```python
from build123d import *

# Parameters (mm, degrees)
F0_R          = 2.3
F1_DEPTH      = 13
F3_DEPTH      = 46
F6_DEPTH      = 52.2
F8_DEPTH      = 25
F10_DEPTH     = 25
F11_T1_DEPTH  = 69.4664340584
F11_T3_DEPTH  = 69.4664340584
F11_T8_DEPTH  = 31.9524083705
F11_T13_DEPTH = 31.9524083705
F11_T19_DEPTH = 31.9524083705
F11_T23_DEPTH = 31.9524083705
F15_DEPTH     = 4
F16_DEPTH     = 4
F19_DEPTH     = 28
F20_R         = 2.3
F21_DEPTH     = 25
F22_R         = 2.3
F23_DEPTH     = 25
F24_R         = 0.5


# Not quite as in the source:
# - a fillet or chamfer that OpenCascade refuses, or shapes differently, is made with other operations: its cross-section is extruded or revolved along the edge and cut away or added
# - a feature names something its author has since deleted; it is built from what else it names


with BuildPart() as f1:
    # F0 (on Front) → F1 (new body)
    with BuildSketch(Plane.XZ):
        Polygon((10, 40), (-10, 40), (-17.9806351662, -11.8325809017), (-8.0368565166, -18.5498173996), (0, -8.6111112242), (8.0368565166, -18.5498173996), (17.9806351662, -11.8325809017), align=None)
        with Locations((-12, 0)):
            Circle(F0_R, mode=Mode.SUBTRACT)
        with Locations((12, 0)):
            Circle(F0_R, mode=Mode.SUBTRACT)
    extrude(amount=-F1_DEPTH)

    # F2 (on face) → F3 (cut)
    with BuildSketch(Plane.XY.offset(40)):
        with BuildLine():
            Line((-8, 0), (8, 0))
            ThreePointArc((8, 0), (0, 8), (-8, 0))
        make_face()
    extrude(amount=-F3_DEPTH, mode=Mode.SUBTRACT)

    # F5 (on offset) → F6 (cut)
    with BuildSketch(Plane.YZ.offset(25)):
        Polygon((13, -3.9485500787), (4.1381944902, -18.5498173996), (13, -18.5498173996), align=None)
    extrude(amount=-F6_DEPTH, mode=Mode.SUBTRACT)

    # F7 (on face) → F8 (cut)
    with BuildSketch(Plane(origin=(-11.122658813, 0, -16.4652915326), x_dir=(0.8286482208, 0, -0.5597697082), z_dir=(-0.5597697082, 0, -0.8286482208))):
        with BuildLine():
            ThreePointArc((-6.8761009811, 0), (-2.2761009811, -4.6), (2.3238990189, 0))
            Line((2.3238990189, 0), (-6.8761009811, 0))
        make_face()
    extrude(amount=-F8_DEPTH, mode=Mode.SUBTRACT)

    # F9 (on face) → F10 (cut)
    with BuildSketch(Plane(origin=(11.122658813, 0, -16.4652915326), x_dir=(0.8286482208, 0, 0.5597697082), z_dir=(0.5597697082, 0, -0.8286482208))):
        with BuildLine():
            ThreePointArc((-2.3238990189, 0), (2.2761009811, -4.6), (6.8761009811, 0))
            Line((6.8761009811, 0), (-2.3238990189, 0))
        make_face()
    extrude(amount=-F10_DEPTH, mode=Mode.SUBTRACT)

    # F11: fillet of radius 5 on 4 edges, made by hand

    # F11_s2 → F11_t1 (cut)
    with BuildSketch(Plane(origin=(7.6867833124, 0, 49.9240736631), x_dir=(0, 1, 0), z_dir=(-0.152176248, 0, -0.9883533728))):
        with BuildLine():
            ThreePointArc((13, -10.9705836466), (11.5355339059, -14.5061175525), (8, -15.9705836466))
            Line((8, -15.9705836466), (13, -15.9705836466))
            Line((13, -15.9705836466), (13, -10.9705836466))
        make_face()
    extrude(amount=F11_T1_DEPTH, mode=Mode.SUBTRACT)

    # F11_s4 → F11_t3 (cut)
    with BuildSketch(Plane(origin=(2.8843579817, 0, -18.733310736), x_dir=(0, 1, 0), z_dir=(-0.152176248, 0, 0.9883533728))):
        with BuildLine():
            ThreePointArc((8, -15.9705836466), (11.5355339059, -14.5061175525), (13, -10.9705836466))
            Line((13, -10.9705836466), (13, -15.9705836466))
            Line((13, -15.9705836466), (8, -15.9705836466))
        make_face()
    extrude(amount=F11_T3_DEPTH, mode=Mode.SUBTRACT)


with BuildPart() as f11_tool6:
    # F11_s7 → F11_t8 (new body)
    with BuildSketch(Plane(origin=(4.0911710208, 3.0705977915, 5.0593097692), x_dir=(0.6002776597, -0.7997916799, 0), z_dir=(-0.5686414, -0.4267895471, -0.7032052622))):
        with BuildLine():
            ThreePointArc((-10.7347001393, -7.9787789452), (-7.9821654916, -9.2854915519), (-4.9822833283, -8.7519638303))
            Line((-4.9822833283, -8.7519638303), (-8.1340389445, -10.4154145762))
            Line((-8.1340389445, -10.4154145762), (-10.7347001393, -7.9787789452))
        make_face()
    extrude(amount=F11_T8_DEPTH)

    split(bisect_by=Plane(origin=(-4.2102294585, 0, -3.404568911), x_dir=(0, 1, 0), z_dir=(-0.7775800359, 0, -0.6287839754)), keep=Keep.TOP)


with BuildPart() as f1_1:
    add(f1.part)

    # F11_t5: cut F11_tool6
    add(f11_tool6.part, mode=Mode.SUBTRACT)


with BuildPart() as f11_tool11:
    # F11_s12 → F11_t13 (new body)
    with BuildSketch(Plane(origin=(14.0782912081, -10.566356105, -17.4097919354), x_dir=(-0.6002776597, -0.7997916799, 0), z_dir=(-0.5686414, 0.4267895471, 0.7032052622))):
        with BuildLine():
            ThreePointArc((-10.7347001393, -7.9787789452), (-7.9821654916, -9.2854915519), (-4.9822833283, -8.7519638303))
            Line((-4.9822833283, -8.7519638303), (-8.1340389445, -10.4154145762))
            Line((-8.1340389445, -10.4154145762), (-10.7347001393, -7.9787789452))
        make_face()
    extrude(amount=F11_T13_DEPTH)

    split(bisect_by=Plane(origin=(4.2102294585, 0, -3.404568911), x_dir=(0, 1, 0), z_dir=(0.7775800359, 0, -0.6287839754)), keep=Keep.TOP)


with BuildPart() as f1_2:
    add(f1_1.part)

    # F11_t10: cut F11_tool11
    add(f11_tool11.part, mode=Mode.SUBTRACT)


with BuildPart() as f11_tool17:
    # F11_s18 → F11_t19 (new body)
    with BuildSketch(Plane(origin=(14.0782912081, -10.566356105, -17.4097919354), x_dir=(-0.6002776597, -0.7997916799, 0), z_dir=(-0.5686414, 0.4267895471, 0.7032052622))):
        with BuildLine():
            ThreePointArc((-10.7347001393, -7.9787789452), (-7.9821654916, -9.2854915519), (-4.9822833283, -8.7519638303))
            Line((-4.9822833283, -8.7519638303), (-8.1340389445, -10.4154145762))
            Line((-8.1340389445, -10.4154145762), (-10.7347001393, -7.9787789452))
        make_face()
    extrude(amount=F11_T19_DEPTH)

    split(bisect_by=Plane(origin=(4.2102294585, 0, -3.404568911), x_dir=(0, 1, 0), z_dir=(-0.7775800359, 0, 0.6287839754)), keep=Keep.TOP)


with BuildPart() as f11_tool21:
    # F11_s22 → F11_t23 (new body)
    with BuildSketch(Plane(origin=(4.0911710208, 3.0705977915, 5.0593097692), x_dir=(0.6002776597, -0.7997916799, 0), z_dir=(-0.5686414, -0.4267895471, -0.7032052622))):
        with BuildLine():
            ThreePointArc((-10.7347001393, -7.9787789452), (-7.9821654916, -9.2854915519), (-4.9822833283, -8.7519638303))
            Line((-4.9822833283, -8.7519638303), (-8.1340389445, -10.4154145762))
            Line((-8.1340389445, -10.4154145762), (-10.7347001393, -7.9787789452))
        make_face()
    extrude(amount=F11_T23_DEPTH)

    split(bisect_by=Plane(origin=(-4.2102294585, 0, -3.404568911), x_dir=(0, 1, 0), z_dir=(0.7775800359, 0, 0.6287839754)), keep=Keep.TOP)


with BuildPart() as f11_tool17_1:
    add(f11_tool17.part)

    # F11_t25: intersect F11_tool21
    add(f11_tool21.part, mode=Mode.INTERSECT)


with BuildPart() as f1_3:
    add(f1_2.part)

    # F11_t15: cut F11_tool17
    add(f11_tool17_1.part, mode=Mode.SUBTRACT)

    # F14 (on face) → F15 (join)
    with BuildSketch(Plane.XZ):
        Polygon((-15.1459260242, -6.5643846345), (-10, 1.0533238305), (-10, 26.8573445146), align=None)
    extrude(amount=F15_DEPTH)

    # F12 (on face) → F16 (join)
    with BuildSketch(Plane.XZ):
        Polygon((15.1459253956, -6.5643830302), (10.0000003771, 26.8573395869), (10.0000003771, 1.0533239459), align=None)
    extrude(amount=F16_DEPTH)

    # F18 (on offset) → F19 (cut)
    with BuildSketch(Plane(origin=(0, 38, 0), x_dir=(-1, 0, 0), z_dir=(0, 1, 0))):
        Polygon((-9.9215390309, 3.6), (-14.0784609691, 3.6), (-16.1569219382, 0), (-14.0784609691, -3.6), (-9.9215390309, -3.6), (-7.8430780618, 0), align=None)
        Polygon((14.0784609691, 3.6), (9.9215390309, 3.6), (7.8430780618, 0), (9.9215390309, -3.6), (14.0784609691, -3.6), (16.1569219382, 0), align=None)
    extrude(amount=-F19_DEPTH, mode=Mode.SUBTRACT)

    # F20 (on face) → F21 (cut)
    with BuildSketch(Plane.XZ.offset(4)):
        with Locations((12, 0)):
            Circle(F20_R)
    extrude(amount=-F21_DEPTH, mode=Mode.SUBTRACT)

    # F22 (on face) → F23 (cut)
    with BuildSketch(Plane.XZ.offset(4)):
        with Locations((-12, 0)):
            Circle(F22_R)
    extrude(amount=-F23_DEPTH, mode=Mode.SUBTRACT)

    # F24
    f24_edges = [f1_3.edges().sort_by_distance(p)[0] for p in [
        (-10, -2, 26.857345),
        (10, -2, 26.85734),
        (-15.145926, -2, -6.564385),
        (15.145925, -2, -6.564383),
        (-10, -2, 1.135782),
        (-13.946588, -2, 1.22507),
        (-14.224942, -2, -0.582781),
        (10, -2, 1.135782),
        (13.946587, -2, 1.22507),
        (14.224941, -2, -0.582782),
        (12.255618, -2, -2.285751),
        (-12.255617, -2, -2.285751),
    ]]
    fillet(f24_edges, radius=F24_R)


solid = f1_3.part
```
Could you check a few things on this model? Use its own coordinates, in mm. A direction names the side the tool comes from. Round coordinates to 2 decimals unless told otherwise and drop trailing zeros. One line per question, with ' | ' between items. Start each with the question number.
(1) Thinking about a two-plate mould opening in Z: for faces 6 (the face through (-2.1, 0, -10.9)), 7 (the face through (3.07, 2.38, -12.41)), 8 (the face through (12, 12, 3.6)), which applies, +Z half, -Z half, draft (parallel to the pull), parting line (faces both ways), or undercut?
(2) For faces 1 (the face through (0, 5, -6)), 2 (the face through (-12, 12, 3.6)), 3 (the face through (14, -4, -3)), 4 (the face through (-3.182, 2.379, -12.546)), 5 (the face through (-13.283, -1.972, -3.806)), which set-ups out of +Z, -Z, +X, -X, +Y, -Y let a thin tool reach every point of the face, with its end or its side?
(3) Please list where these lines run through material, in increasing order: line 1 along X through (y, z) = (1.5, 0); line 2 along X through (y, z) = (5.5, 0); line 3 along Y through (x, z) = (0, 18).
(4) For P1, Ø2, axis at y = 3.5, z = -10, coming from the -X side; P2, Ø6.5, axis at x = -3.5, z = -13, coming from the -Y side; P3, Ø6, axis at x = -12, z = 0, coming from the +Y side, each with a flat end and sliding along its axis, tell me the tip position at first contact or that it passes through.
(5) Suppose I cut it at A-A on y = 3.25. Count the separate pieces of the cut face and the enclosed holes in it, then the cut area to 3 significant figures.
Geometry results:
1) face 6: draft | face 7: -Z half | face 8: undercut
2) face 1: +Z, -Y | face 2: +Y | face 3: +Z, -Z, +X, -X, -Y | face 4: -Z, +Y, -Y | face 5: -Z, -Y
3) line 1: -16.16 to -14.3, -9.7 to -7.99, 7.99 to 9.7, 14.3 to 16.16 | line 2: -16.16 to -14.3, -9.7 to -5.81, 5.81 to 9.7, 14.3 to 16.16 | line 3: 8 to 13
4) P1: x = -17.85 | P2: y = 0 | P3: y = 10
5) separate pieces: 3 | enclosed holes: 2 | area: 674 mm²
